from build123d import *

# Parameters (mm, degrees)
SKETCH1_W           = 35
SKETCH1_H           = 35
SKETCH1_R           = 5
BOSS_EXTRUDE1_DEPTH = 15
SKETCH2_R           = 1.75
CUT_EXTRUDE1_DEPTH  = 10
CHAMFER1_SIZE       = 1
SKETCH3_R           = 2
CUT_EXTRUDE2_DEPTH  = 10


with BuildPart() as part:
    # Sketch1 → Boss-Extrude1 (new body, symmetric)
    with BuildSketch(Plane.XY):
        with Locations((0, 1.5)):
            Rectangle(SKETCH1_W, SKETCH1_H)
        with Locations((0, 1.5)):
            Circle(SKETCH1_R, mode=Mode.SUBTRACT)
    extrude(amount=BOSS_EXTRUDE1_DEPTH, both=True)

    # Sketch2 → Cut-Extrude1 (cut)
    with BuildSketch(Plane.XY.offset(15)):
        with Locations((0, 9.5)):
            Circle(SKETCH2_R)
        with Locations((0, -6.5)):
            Circle(SKETCH2_R)
        with Locations((8, 1.5)):
            Circle(SKETCH2_R)
        with Locations((-8, 1.5)):
            Circle(SKETCH2_R)
    extrude(amount=-CUT_EXTRUDE1_DEPTH, mode=Mode.SUBTRACT)

    # Chamfer1
    chamfer1_edges = [part.edges().sort_by_distance(p)[0] for p in [
        (-17.5, 19, 0),
        (17.5, 19, 0),
        (17.5, -16, 0),
        (-17.5, -16, 0),
    ]]
    chamfer(chamfer1_edges, length=CHAMFER1_SIZE)

    # Sketch3 → Cut-Extrude2 (cut)
    with BuildSketch(Plane.XZ.offset(16)):
        with Locations((12.5, 8)):
            Circle(SKETCH3_R)
        with Locations((12.5, -8)):
            Circle(SKETCH3_R)
    cut_extrude2 = extrude(amount=-CUT_EXTRUDE2_DEPTH, mode=Mode.SUBTRACT)

    # Mirror1: Cut-Extrude2 across plane
    add(cut_extrude2.mirror(Plane(origin=(0, 0, 0), x_dir=(0, 0, 1), z_dir=(1, 0, 0))), mode=Mode.SUBTRACT)


solid = part.part
Source: CAD feature listing. Evaluate the final solid. Frame: model axes, mm. A direction names the side the tool comes from. Coordinates: 2 decimals unless noted, no trailing zeros. Loops run counter-clockwise (first coordinate to the right, second up) from the corner with the lowest first, then second, coordinate; pieces in that order, holes last. Notation, with made-up numbers: (85.25, 50) -> (144.25, 50) arc R19 ccw to (144.25, 68) -> close; hole circle Ø3 at (63.25, -37). An arc over 180 degrees is marked (long way). Answer in a Markdown table with one row per item. Add a question column.
Q1. Section A-A on x = -4. Return the cut outline in (y, z).
Q2. Ray query, line 1 along Y through (x, z) = (-8, 7.5); line 2 along Y through (x, z) = (1.5, 7.75); line 3 along Z through (x, y) = (9, 2). Return the intervals inside material, ascending.
Q3. Section D-D on y = -13.5. Return the cut outline in (x, z).
Q4. Contact query for flat-ended pins moving along their axis: pin 1 Ø1.8 at (x, y) = (-8, 1) entering from +Z; pin 2 Ø1.2 at (x, z) = (13, -8.5) entering from -Y. Output: stop coordinate, or through.
Q5. Section C-C on y = 5.5. Return the cut outline in (x, z), and give its area (3 significant figures).
Q6. Section B-B on z = -4.5. Return the cut outline in (x, y), and give its area (3 significant figures).
Q7. Pull-direction query (X, two-part tool) for faces 1 (the face through (17, -15.5, -0.2)), 2 (the face through (-17, 18.5, 0.2)), 3 (the face through (12, -6, -8)); classes: pulls with the +X half, pulls with the -X half, needs draft (parallel to the pull), parting line crosses it, or undercut.
Q8. Reachability of faces 4 (the face through (8, 2, 5)), 5 (the face through (-12, -6, -8)), 6 (the face through (4, 6, 15)) from +Z, -Z, +X, -X, +Y, -Y: full face, straight path, thin tool, end or side. Return the list, or none.
Computed values:
| question | item | result |
|---|---|---|
| 1 | outline | (-16, -15) -> (-1.5, -15) -> (-1.5, 15) -> (-16, 15) -> close; (4.5, -15) -> (19, -15) -> (19, 15) -> (4.5, 15) -> close |
| 2 | line 1 | y = -16 to -0.25, 3.25 to 19 |
| 2 | line 2 | y = -16 to -7.4, -5.6 to -3.27, 6.27 to 8.6, 10.4 to 19 |
| 2 | line 3 | z = -15 to 5 |
| 3 | outline | (-17.5, -15) -> (17.5, -15) -> (17.5, 15) -> (-17.5, 15) -> close; hole circle Ø4 at (-12.5, -8); hole circle Ø4 at (-12.5, 8); hole circle Ø4 at (12.5, -8); hole circle Ø4 at (12.5, 8) |
| 4 | pin 1 | stops at z = 5 |
| 4 | pin 2 | stops at y = -6 |
| 5 | outline | (-17.5, -15) -> (-3, -15) -> (-3, 15) -> (-17.5, 15) -> close; (3, -15) -> (17.5, -15) -> (17.5, 15) -> (3, 15) -> close |
| 5 | area | 870 mm^2 |
| 6 | outline | (-17.5, -15) -> (-16.5, -16) -> (16.5, -16) -> (17.5, -15) -> (17.5, 18) -> (16.5, 19) -> (-16.5, 19) -> (-17.5, 18) -> close; hole circle Ø10 at (0, 1.5) |
| 6 | area | 1,140 mm^2 |
| 7 | face 1 | pulls with the +X half |
| 7 | face 2 | pulls with the -X half |
| 7 | face 3 | undercut |
| 8 | face 4 | +Z |
| 8 | face 5 | -Y |
| 8 | face 6 | +Z, +X, -X, +Y, -Y |
